Input: part model. Units: mm. Frame: model coordinates. A direction names the side the tool comes from. Give positions to 0.01 mm unless a question says otherwise; leave off trailing zeros. Write each loop counter-clockwise with the first axis right and the second up, starting at its lowest first coordinate (ties: lowest second). Pieces come first, ordered by that corner, then holes. Notation, with made-up numbers: (-24.5, 3.25) - (11.5, 3.25) arc R23 ccw to (11.5, 17.25) - close; hole circle Ø4 at (-15.75, 48.5). An arc over 180 degrees is marked (long way). Answer as CSV lines item,"result". Start each with the question number.
from build123d import *

# Parameters (mm, degrees)
ESQUISSE1_R                = 1.5
BOSS_EXTRU_1_DEPTH         = 3
ESQUISSE2_R                = 1.5
BOSS_EXTRU_2_DEPTH         = 10
R_P_TITION_LIN_AIRE1_COUNT = 2
R_P_TITION_LIN_AIRE1_PITCH = 20


with BuildPart() as part:
    # Esquisse1 → Boss.-Extru.1 (new body)
    with BuildSketch(Plane.XY):
        with BuildLine():
            Line((-15, 7.5), (15, 7.5))
            ThreePointArc((15, 7.5), (18.535533906, 6.035533906), (20, 2.5))
            Line((20, 2.5), (20, -7.5))
            Line((20, -7.5), (-20, -7.5))
            Line((-20, -7.5), (-20, 2.5))
            ThreePointArc((-20, 2.5), (-18.535533906, 6.035533906), (-15, 7.5))
        make_face()
        with Locations((-15, -2.5)):
            Circle(ESQUISSE1_R, mode=Mode.SUBTRACT)
        with Locations(Location((15, -2.5, 0), (0, 0, 180))):
            Circle(ESQUISSE1_R, mode=Mode.SUBTRACT)
        with Locations((0, 2.5)):
            Circle(ESQUISSE1_R, mode=Mode.SUBTRACT)
    extrude(amount=BOSS_EXTRU_1_DEPTH)

    # Esquisse2 → Boss.-Extru.2 (add)
    with BuildSketch(Plane(origin=(20, 0, 0), x_dir=(0, 0, -1), z_dir=(1, 0, 0))):
        with BuildLine():
            Line((-0.009486275, -9.782419246), (0, -7.5))
            Line((0, -7.5), (-2.5, -7.5))
            Line((-2.5, -7.5), (-3, -7.5))
            Line((-3, -7.5), (-3, -7.550510257))
            ThreePointArc((-3, -7.550510257), (-3.995289489, -12.003524231), (-0.009486275, -9.782419246))
        make_face()
        with Locations((-2.5, -10)):
            Circle(ESQUISSE2_R, mode=Mode.SUBTRACT)
    boss_extru_2 = extrude(amount=-BOSS_EXTRU_2_DEPTH)

    # Répétition linéaire1: Boss.-Extru.2 ×2
    with Locations(*[(-i * R_P_TITION_LIN_AIRE1_PITCH, 0, 0) for i in range(1, R_P_TITION_LIN_AIRE1_COUNT)]):
        add(boss_extru_2)


solid = part.part
1) Material intervals for line 1 (Y direction, x = 15, z = 2.5); line 2 (Y direction, x = 15, z = 1.8); line 3 (X direction, y = -3.5, z = 0.5), sorted ascending. Write a range as from..to.
2) Reachability of faces 1 (the flat face through (0, 0, 3)), 2 (the flat face through (-10, -9, 1)), 3 (the flat face through (5, -7.5, 1)), 4 (the cylindrical face through (18.5, 6.07, 1.48)) from +Z, -Z, +X, -X, +Y, -Y: full face, straight path, thin tool, end or side. Return the list, or none.
3) Contact query for flat-ended pins moving along their axis: P1, Ø1, axis at y = 5, z = 3, coming from the -X side; P2, Ø2.5, axis at x = 0, y = 2.5, coming from the -Z side; P3, Ø1.5, axis at y = -9, z = 3, coming from the -X side; P4, Ø0.9, axis at x = -17, z = 1, coming from the -Y side. Output: stop coordinate, or through.
4) Cut plane B-B on x = 14. Output: boundary loops of the cut face in (y, z).
5) Pull-direction query (Z, two-part tool) for faces 5 (the cylindrical face through (15, -12, 4)), 6 (the cylindrical face through (-4.93, -11.464, 2.825)), 7 (the flat face through (-15, -7.5, 1)); classes: +Z half, -Z half, draft (parallel to the pull), parting line (faces both ways), or undercut.
6) Cut plane A-A on z = 2.5. Output: boundary loops of the cut face in (x, y), and give its area (3 significant figures).
7) Cut plane D-D on z = 0.5. Output: boundary loops of the cut face in (x, y).
8) Cut plane C-C on y = -2.5. Output: boundary loops of the cut face in (x, z).
Numbers:
1,line 1,"y = -12.5..-11.5, -8.5..-4, -1..7.5"
1,line 2,"y = -12.4..-11.33, -8.67..-4, -1..7.5"
1,line 3,"x = -20..-16.12, -13.88..13.88, 16.12..20"
2,face 1,"+Z, +X, -X, +Y"
2,face 2,"+Z, -Z, -X, -Y"
2,face 3,"+Z, -Z, -Y"
2,face 4,"+Z, -Z, +X, +Y"
3,P1,"stops at x = -19.58"
3,P2,"passes through"
3,P3,"stops at x = -10"
3,P4,"stops at y = -7.5"
4,outline,"(-9.78, 0.01) - (-7.5, 0) - (-3.62, 0) - (-3.62, 3) - (-7.55, 3) arc R2.5 ccw (long way) to start; (-1.38, 0) - (7.5, 0) - (7.5, 3) - (-1.38, 3) - close; hole circle Ø3 at (-10, 2.5)"
5,face 5,"parting line"
5,face 6,"undercut"
5,face 7,"draft"
6,outline,"(-20, -7.5) - (-10, -7.5) - (-10, -8.5) - (0, -8.5) - (0, -7.5) - (10, -7.5) - (10, -8.5) - (20, -8.5) - (20, 2.5) arc R5 ccw to (15, 7.5) - (-15, 7.5) arc R5 ccw to (-20, 2.5) - close; (-10, -12.5) - (0, -12.5) - (0, -11.5) - (-10, -11.5) - close; (10, -12.5) - (20, -12.5) - (20, -11.5) - (10, -11.5) - close; hole circle Ø3 at (-15, -2.5); hole circle Ø3 at (0, 2.5); hole circle Ø3 at (15, -2.5)"
6,area,"608 mm²"
7,outline,"(-20, -7.5) - (-10, -7.5) - (-10, -11.5) - (0, -11.5) - (0, -7.5) - (10, -7.5) - (10, -11.5) - (20, -11.5) - (20, 2.5) arc R5 ccw to (15, 7.5) - (-15, 7.5) arc R5 ccw to (-20, 2.5) - close; hole circle Ø3 at (-15, -2.5); hole circle Ø3 at (0, 2.5); hole circle Ø3 at (15, -2.5)"
8,outline,"(-20, 0) - (-16.5, 0) - (-16.5, 3) - (-20, 3) - close; (-13.5, 0) - (13.5, 0) - (13.5, 3) - (-13.5, 3) - close; (16.5, 0) - (20, 0) - (20, 3) - (16.5, 3) - close"
